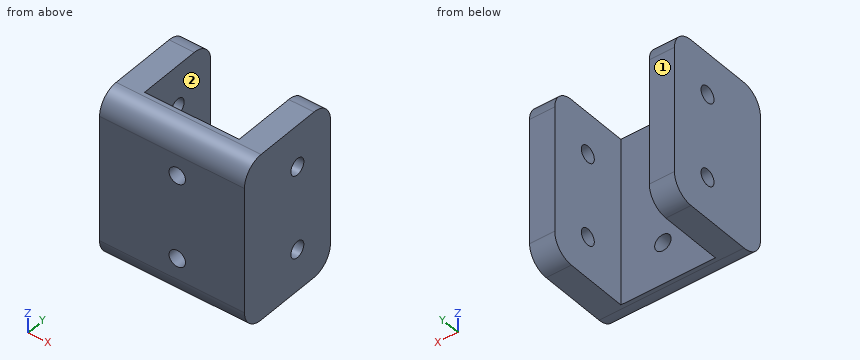
```python
from build123d import *

# Parameters (mm, degrees)
BOSS_EXTRUDE1_DEPTH = 50.8
FILLET1_R           = 6.35
SKETCH2_R           = 2.4892
CUT_EXTRUDE1_DEPTH  = 75.771081475
SKETCH3_R           = 2.4892
CUT_EXTRUDE2_DEPTH  = 75.771081475


with BuildPart() as part:
    # Sketch1 → Boss-Extrude1 (new body)
    with BuildSketch(Plane.XY):
        Polygon((0, 33.02), (0, 0), (43.815, 0), (43.815, 33.02), (36.195, 33.02), (36.195, 7.62), (7.62, 7.62), (7.62, 33.02), align=None)
    extrude(amount=-BOSS_EXTRUDE1_DEPTH)

    # Fillet1
    fillet1_edges = [part.edges().sort_by_distance(p)[0] for p in [
        (21.9075, 0, 0),
        (3.81, 33.02, 0),
        (40.005, 33.02, 0),
        (3.81, 33.02, -50.8),
        (21.9075, 0, -50.8),
        (40.005, 33.02, -50.8),
    ]]
    fillet(fillet1_edges, radius=FILLET1_R)

    # Sketch2 → Cut-Extrude1 (cut, through all)
    with BuildSketch(Plane.ZY):
        with Locations((-38.1, 20.32)):
            Circle(SKETCH2_R)
        with Locations((-12.7, 20.32)):
            Circle(SKETCH2_R)
    extrude(amount=-CUT_EXTRUDE1_DEPTH, mode=Mode.SUBTRACT)

    # Sketch3 → Cut-Extrude2 (cut, through all)
    with BuildSketch(Plane.XZ):
        with Locations(Location((23.495, -38.1, 0), (0, 0, 270))):
            Circle(SKETCH3_R)
        with Locations(Location((23.495, -12.7, 0), (0, 0, 270))):
            Circle(SKETCH3_R)
    extrude(amount=-CUT_EXTRUDE2_DEPTH, mode=Mode.SUBTRACT)


solid = part.part
```
The model under review builds one solid part; all positions refer to its coordinate system, in mm. Face numbers are marked on the shaded views. A direction names the side the tool comes from. Round coordinates to 2 decimals unless told otherwise and drop trailing zeros. Order: outer loops, then holes, each group sorted by start corner. A loop starts at its lowest first (then second) coordinate and runs counter-clockwise, first axis right, second up.
(1) For P1, Ø1.5, axis at y = 25, z = -31.5, coming from the -X side; P2, Ø6, axis at x = 12, z = -25, coming from the +Y side, all flat-tipped, find the tip position at first contact; note any pin that passes through.
Working result:
P1: stops at x = 0
P2: stops at y = 7.62
(2) Take a section at B-B, the plane x = 5. State the section outline as (y, z) points.
Working result:
outline: (0, -44.45) arc R6.35 ccw to (6.35, -50.8) - (26.67, -50.8) arc R6.35 ccw to (33.02, -44.45) - (33.02, -6.35) arc R6.35 ccw to (26.67, 0) - (6.35, 0) arc R6.35 ccw to (0, -6.35) - close; hole circle Ø4.98 at (20.32, -38.1); hole circle Ø4.98 at (20.32, -12.7)
(3) Wall thickness on L1, parallel to X at y = 15, z = -21 (3 decimals); L2, parallel to Y at x = 3, z = -12.7; L3, parallel to Y at x = 9.5, z = -16: over which ranges is each line inside the solid? List them lowest first.
Working result:
L1: x = 0 to 7.62, 36.195 to 43.815
L2: y = 0 to 17.83, 22.81 to 33.02
L3: y = 0 to 7.62
(4) Take a section at A-A, the plane y = 15. State the section outline as (x, z) points (3 decimals), plus the area to 3 significant figures.
Working result:
outline: (0, -50.8) - (7.62, -50.8) - (7.62, 0) - (0, 0) - close; (36.195, -50.8) - (43.815, -50.8) - (43.815, 0) - (36.195, 0) - close
area: 774 mm2
(5) Take a section at C-C, the plane z = -12.7. State the section outline as (x, y) points (3 decimals), plus the area to 3 significant figures.
Working result:
outline: (0, 0) - (21.006, 0) - (21.006, 7.62) - (7.62, 7.62) - (7.62, 17.831) - (0, 17.831) - close; (0, 22.809) - (7.62, 22.809) - (7.62, 33.02) - (0, 33.02) - close; (25.984, 0) - (43.815, 0) - (43.815, 17.831) - (36.195, 17.831) - (36.195, 7.62) - (25.984, 7.62) - close; (36.195, 22.809) - (43.815, 22.809) - (43.815, 33.02) - (36.195, 33.02) - close
area: 607 mm2
(6) Take a section at D-D, the plane y = 20.32. State the section outline as (x, z) points (3 decimals).
Working result:
outline: (0, -50.8) - (7.62, -50.8) - (7.62, -40.589) - (0, -40.589) - close; (0, -35.611) - (7.62, -35.611) - (7.62, -15.189) - (0, -15.189) - close; (0, -10.211) - (7.62, -10.211) - (7.62, 0) - (0, 0) - close; (36.195, -50.8) - (43.815, -50.8) - (43.815, -40.589) - (36.195, -40.589) - close; (36.195, -35.611) - (43.815, -35.611) - (43.815, -15.189) - (36.195, -15.189) - close; (36.195, -10.211) - (43.815, -10.211) - (43.815, 0) - (36.195, 0) - close
(7) Tool access review of the marked faces 1 and 2: name each direction out of +Z, -Z, +X, -X, +Y, -Y from which nothing blocks a thin tool from reaching the whole face with its end or side.
Working result:
face 1: +Z, -Z, +X, -X, +Y
face 2: +Z, -Z, +Y
